Check sheet for the modelled part. Datum: model origin and axes. Units: mm. Face numbers are marked on the shaded views. A direction names the side the tool comes from. Round coordinates to 2 decimals unless told otherwise and drop trailing zeros. Write each loop counter-clockwise with the first axis right and the second up, starting at its lowest first coordinate (ties: lowest second). Pieces come first, ordered by that corner, then holes. Notation, with made-up numbers: (82, 20.5) - (119, 20.5) arc R22 ccw to (119, 29.5) - close; hole circle Ø8 at (-3.5, 30.25). An arc over 180 degrees is marked (long way). Answer as a JSON object with one key per item and string values. Group by question number.
Item 1: Release check for a two-part mould opening along Y. For the marked faces 4, 5 and 6 record: pulls with the +Y half, pulls with the -Y half, needs draft (parallel to the pull), parting line crosses it, or undercut.
Item 2: Sectioned sample at B-B on x = 0. Count the separate pieces of the cut face and the enclosed holes in it, plus the area to 3 significant figures.
Item 3: Sectioned sample at D-D on z = 5.5. Record the boundary of the cut face in (x, y).
Item 4: Thickness scan on line 1 (Y direction, x = 10.5, z = -20.5); line 2 (Y direction, x = 16.5, z = -6); line 3 (X direction, y = 14.5, z = 6.5). Record the ranges inside material, lowest first.
Item 5: Sectioned sample at A-A on y = 22.4. Record the boundary of the cut face in (x, z).
Item 6: Set-up check for the marked faces 1, 2 and 3: record each of +Z, -Z, +X, -X, +Y, -Y from which the full face is reachable in a straight line by a thin tool's end or side.
Item 7: Sectioned sample at C-C on y = 18.5. Record the boundary of the cut face in (x, z), plus the area to 3 significant figures.
Item 8: Gauge pin test, flat ends, axial feed: P1, Ø12, axis at y = -3.5, z = -3, coming from the -X side; P2, Ø4.5, axis at y = 22.4, z = -6, coming from the +X side; P3, Ø1.3, axis at x = 6, y = 15.5, coming from the +Z side; P4, Ø7.5, axis at y = 14, z = 6.5, coming from the -X side. Record the tip position at first contact, or that the pin passes through.
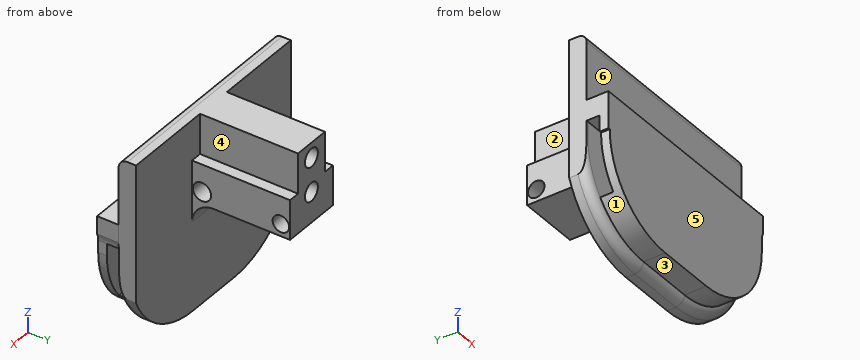
```python
from build123d import *

# Parameters (mm, degrees)
SALIENTE_EXTRUIR1_DEPTH     = 2
SALIENTE_EXTRUIR2_DEPTH     = 24.5
SALIENTE_EXTRUIR3_DEPTH     = 22.5
CORTAR_EXTRUIR1_DEPTH       = 27
CORTAR_EXTRUIR1_DEPTH_BACK  = 65.5
CROQUIS4_R                  = 1.599999999
REDONDEO1_R                 = 3
REDONDEO2_R                 = 5
SALIENTE_EXTRUIR5_START     = 2
SALIENTE_EXTRUIR5_DEPTH     = 2
CROQUIS16_W                 = 2.6
CROQUIS16_H                 = 16.420237112
CORTAR_EXTRUIR8_DEPTH       = 22.5
REDONDEO6_R                 = 2
REDONDEO7_R                 = 2
CROQUIS5_R                  = 2.1
CORTAR_EXTRUIR2_DEPTH       = 20.5
CROQUIS17_R                 = 2.1
CORTAR_EXTRUIR9_DEPTH       = 10
CORTAR_EXTRUIR14_DEPTH      = 11
CORTAR_EXTRUIR14_DEPTH_BACK = 10
CROQUIS18_R                 = 1.9
CROQUIS19_R                 = 18.5
CORTAR_EXTRUIR15_DEPTH      = 3.5
CORTAR_EXTRUIR16_START      = -56
CROQUIS20_R                 = 18.5
CORTAR_EXTRUIR16_DEPTH      = 3.5
CROQUIS21_W                 = 93.525691526
CROQUIS21_H                 = 152.705287602
CROQUIS21_W_2               = 50.201984064
CROQUIS21_H_2               = 74.038187446
CORTAR_EXTRUIR17_DEPTH      = 79
SALIENTE_EXTRUIR6_DEPTH     = 5
CROQUIS23_W                 = 15
CROQUIS23_H                 = 3
CORTAR_EXTRUIR18_DEPTH      = 87


# Read off the part's stored shape, not the designer's step: Saliente-Extruir6
with BuildPart() as part:
    # Croquis1 → Saliente-Extruir1 (new body)
    with BuildSketch(Plane(origin=(0, 0, 0), x_dir=(1, 0, 0), z_dir=(0, 1, 0))):
        with BuildLine():
            Line((-31.5, -9.464532567), (31.5, -9.464532567))
            Line((31.5, -9.464532567), (31.5, 7.964532567))
            ThreePointArc((31.5, 7.964532567), (31.060660172, 9.025192739), (30, 9.464532567))
            Line((30, 9.464532567), (28.160101256, 9.464532567))
            ThreePointArc((28.160101256, 9.464532567), (27.099441084, 9.903872396), (26.660101256, 10.964532567))
            Line((26.660101256, 10.964532567), (26.660101256, 14.266885585))
            ThreePointArc((26.660101256, 14.266885585), (20.802236879, 28.409021208), (6.660101256, 34.266885585))
            Line((6.660101256, 34.266885585), (-6.660101256, 34.266885585))
            ThreePointArc((-6.660101256, 34.266885585), (-20.802236879, 28.409021208), (-26.660101256, 14.266885585))
            Line((-26.660101256, 14.266885585), (-26.660101256, 10.964532567))
            ThreePointArc((-26.660101256, 10.964532567), (-27.099441084, 9.903872396), (-28.160101256, 9.464532567))
            Line((-28.160101256, 9.464532567), (-30, 9.464532567))
            ThreePointArc((-30, 9.464532567), (-31.060660172, 9.025192739), (-31.5, 7.964532567))
            Line((-31.5, 7.964532567), (-31.5, -9.464532567))
        make_face()
    extrude(amount=SALIENTE_EXTRUIR1_DEPTH)

    # Croquis2 → Saliente-Extruir2 (add)
    with BuildSketch(Plane(origin=(0, 0, 0), x_dir=(1, 0, 0), z_dir=(0, 1, 0))):
        Polygon((6.95, -8.819174125), (6.95, -9.464532567), (-6.95, -9.464532567), (-6.95, -8.819174125), (-6.95, 8.819174125), (6.95, 8.819174125), align=None)
    extrude(amount=SALIENTE_EXTRUIR2_DEPTH)

    # Croquis3 → Saliente-Extruir3 (add)
    with BuildSketch(Plane(origin=(0, 2, 0), x_dir=(1, 0, 0), z_dir=(0, 1, 0))):
        with BuildLine():
            ThreePointArc((28.160101256, 9.464532567), (27.375457574, 9.686121721), (26.822638598, 10.285420177))
            Line((26.822638598, 10.285420177), (25.6, 10.285420177))
            Line((25.6, 10.285420177), (25.6, -2.749999823))
            Line((25.6, -2.749999823), (31.5, -2.749999823))
            Line((31.5, -2.749999823), (31.5, 7.964532567))
            ThreePointArc((31.5, 7.964532567), (31.060660172, 9.025192739), (30, 9.464532567))
            Line((30, 9.464532567), (28.160101256, 9.464532567))
        make_face()
        with BuildLine():
            Line((-25.6, 10.285420177), (-26.822638598, 10.285420177))
            ThreePointArc((-26.822638598, 10.285420177), (-27.375457574, 9.686121721), (-28.160101256, 9.464532567))
            Line((-28.160101256, 9.464532567), (-30, 9.464532567))
            ThreePointArc((-30, 9.464532567), (-31.060660172, 9.025192739), (-31.5, 7.964532567))
            Line((-31.5, 7.964532567), (-31.5, -2.749999823))
            Line((-31.5, -2.749999823), (-25.6, -2.749999823))
            Line((-25.6, -2.749999823), (-25.6, 10.285420177))
        make_face()
    extrude(amount=SALIENTE_EXTRUIR3_DEPTH)

    # Croquis4 → Cortar-Extruir1 (cut, two sides: drawn at the far end of the back side and taken through both)
    with BuildSketch(Plane.ZY.offset(25.5).offset(-CORTAR_EXTRUIR1_DEPTH_BACK)):
        with Locations((-6.002353017, 4.3)):
            Circle(CROQUIS4_R)
        with Locations((-6.002353017, 22.4)):
            Circle(CROQUIS4_R)
    extrude(amount=CORTAR_EXTRUIR1_DEPTH + CORTAR_EXTRUIR1_DEPTH_BACK, mode=Mode.SUBTRACT)

    # Redondeo1
    redondeo1_edges = [part.edges().sort_by_distance(p)[0] for p in [
        (28.55, 2, 2.749999823),
    ]]
    fillet(redondeo1_edges, radius=REDONDEO1_R)

    # Redondeo2
    redondeo2_edges = [part.edges().sort_by_distance(p)[0] for p in [
        (0, 2, -8.819174125),
    ]]
    fillet(redondeo2_edges, radius=REDONDEO2_R)

    # Croquis15 → Saliente-Extruir5 (add)
    with BuildSketch(Plane.XZ.offset(SALIENTE_EXTRUIR5_START)):
        with BuildLine():
            Line((-31.5, 9.464532567), (31.5, 9.464532567))
            Line((31.5, 9.464532567), (31.5, -7.489095092))
            ThreePointArc((31.5, -7.489095092), (30.914213562, -8.903308654), (29.5, -9.489095092))
            Line((29.5, -9.489095092), (28.660101256, -9.489095092))
            ThreePointArc((28.660101256, -9.489095092), (27.245887693, -10.074881529), (26.660101256, -11.489095092))
            Line((26.660101256, -11.489095092), (26.660101256, -14.266885585))
            ThreePointArc((26.660101256, -14.266885585), (20.802236879, -28.409021208), (6.660101256, -34.266885585))
            Line((6.660101256, -34.266885585), (1.137553535, -34.266885585))
            Line((1.137553535, -34.266885585), (-1.137553535, -34.266885585))
            Line((-1.137553535, -34.266885585), (-6.660101256, -34.266885585))
            ThreePointArc((-6.660101256, -34.266885585), (-20.802236879, -28.409021208), (-26.660101256, -14.266885585))
            Line((-26.660101256, -14.266885585), (-26.660101256, -11.489095092))
            ThreePointArc((-26.660101256, -11.489095092), (-27.245887693, -10.074881529), (-28.660101256, -9.489095092))
            Line((-28.660101256, -9.489095092), (-29.5, -9.489095092))
            ThreePointArc((-29.5, -9.489095092), (-30.914213562, -8.903308654), (-31.5, -7.489095092))
            Line((-31.5, -7.489095092), (-31.5, 9.464532567))
        make_face()
    extrude(amount=-SALIENTE_EXTRUIR5_DEPTH)

    # Croquis16 → Cortar-Extruir8 (cut)
    with BuildSketch(Plane(origin=(0, 24.5, 0), x_dir=(1, 0, 0), z_dir=(0, 1, 0))):
        with Locations((5.65, -8.484535845)):
            Rectangle(CROQUIS16_W, CROQUIS16_H)
        with Locations((-5.65, -8.484535845)):
            Rectangle(CROQUIS16_W, CROQUIS16_H)
    extrude(amount=-CORTAR_EXTRUIR8_DEPTH, mode=Mode.SUBTRACT)

    # Redondeo6
    redondeo6_edges = [part.edges().sort_by_distance(p)[0] for p in [
        (-31.5, -2, 0.987718738),
        (-30.914213562, -2, -8.903308654),
        (-29.080050628, -2, -9.489095092),
        (-27.245887693, -2, -10.074881529),
        (-26.660101256, -2, -12.877990338),
        (-20.802236879, -2, -28.409021208),
        (0, -2, -34.266885585),
        (20.802236879, -2, -28.409021208),
        (26.660101256, -2, -12.877990338),
        (27.245887693, -2, -10.074881529),
        (29.080050628, -2, -9.489095092),
        (30.914213562, -2, -8.903308654),
        (31.5, -2, 0.987718738),
    ]]
    fillet(redondeo6_edges, radius=REDONDEO6_R - 0.0001)  # a hair under: the kernel refuses the full size

    # Redondeo7
    redondeo7_edges = [part.edges().sort_by_distance(p)[0] for p in [
        (0, -2, 9.464532567),
        (30.914242852, -1.414242852, 9.464532567),
        (-30.914242852, -1.414242852, 9.464532567),
        (31.5, 0.99995, 9.464532567),
        (-31.5, 0.99995, 9.464532567),
    ]]
    fillet(redondeo7_edges, radius=REDONDEO7_R - 0.0001)  # a hair under: the kernel refuses the full size

    # Croquis5 → Cortar-Extruir2 (cut)
    with BuildSketch(Plane(origin=(0, 24.5, 0), x_dir=(1, 0, 0), z_dir=(0, 1, 0))):
        with Locations(Location((0, 1.798301608, 0), (0, 0, 270))):
            Circle(CROQUIS5_R)
        with Locations(Location((0, -6.026932469, 0), (0, 0, 270))):
            Circle(CROQUIS5_R)
        with Locations(Location((-28.55, 1.798301608, 0), (0, 0, 270))):
            Circle(CROQUIS5_R)
        with Locations(Location((28.55, 1.798301608, 0), (0, 0, 270))):
            Circle(CROQUIS5_R)
    extrude(amount=-CORTAR_EXTRUIR2_DEPTH, mode=Mode.SUBTRACT)

    # Croquis17 → Cortar-Extruir9 (cut, symmetric)
    with BuildSketch(Plane(origin=(0, 0, 0), x_dir=(0, 0, -1), z_dir=(1, 0, 0))):
        with Locations((6.002353017, 4.3)):
            Circle(CROQUIS17_R)
    extrude(amount=CORTAR_EXTRUIR9_DEPTH, both=True, mode=Mode.SUBTRACT)

    # Croquis18 → Cortar-Extruir14 (cut, two sides: drawn at the far end of the back side and taken through both)
    with BuildSketch(Plane(origin=(0, 0, 0), x_dir=(0, 0, -1), z_dir=(1, 0, 0)).offset(-CORTAR_EXTRUIR14_DEPTH_BACK)):
        with Locations(Location((6.002353017, 22.4, 0), (0, 0, 180))):
            Circle(CROQUIS18_R)
    extrude(amount=CORTAR_EXTRUIR14_DEPTH + CORTAR_EXTRUIR14_DEPTH_BACK, mode=Mode.SUBTRACT)

    # Croquis19 → Cortar-Extruir15 (cut)
    with BuildSketch(Plane(origin=(31.5, 0, 0), x_dir=(0, 0, -1), z_dir=(1, 0, 0))):
        with Locations((25.179802512, 14.045485316)):
            Circle(CROQUIS19_R)
    extrude(amount=-CORTAR_EXTRUIR15_DEPTH, mode=Mode.SUBTRACT)

    # Croquis20 → Cortar-Extruir16 (cut)
    with BuildSketch(Plane(origin=(28, 0, 0), x_dir=(0, 0, -1), z_dir=(1, 0, 0)).offset(CORTAR_EXTRUIR16_START)):
        with Locations((25.179802512, 14.045485316)):
            Circle(CROQUIS20_R)
    extrude(amount=-CORTAR_EXTRUIR16_DEPTH, mode=Mode.SUBTRACT)

    # Croquis21 → Cortar-Extruir17 (cut)
    with BuildSketch(Plane(origin=(0, 24.5, 0), x_dir=(1, 0, 0), z_dir=(0, 1, 0))):
        Rectangle(CROQUIS21_W, CROQUIS21_H)
        Rectangle(CROQUIS21_W_2, CROQUIS21_H_2, mode=Mode.SUBTRACT)
    extrude(amount=-CORTAR_EXTRUIR17_DEPTH, mode=Mode.SUBTRACT)

    # Saliente-Extruir6 outline → Saliente-Extruir6 (add)
    with BuildSketch(Plane.XZ.offset(2)):
        with BuildLine():
            Line((25.004354391, -5.79015449), (-25.100992032, -5.79015449))
            Line((-25.100992032, -5.79015449), (-25.100992032, -14.266885585))
            Line((-25.100992032, -14.266885585), (-24.660101256, -14.266885585))
            ThreePointArc((-24.660101256, -14.266885585), (-19.388023317, -26.994807646), (-6.660101256, -32.266885585))
            Line((-6.660101256, -32.266885585), (6.660101256, -32.266885585))
            ThreePointArc((6.660101256, -32.266885585), (19.388023317, -26.994807646), (24.660101256, -14.266885585))
            Line((24.660101256, -14.266885585), (24.660101256, -11.489095092))
            ThreePointArc((24.660101256, -11.489095092), (24.747110874, -10.659332312), (25.004354391, -9.865668204))
            Line((25.004354391, -9.865668204), (25.004354391, -5.79015449))
        make_face()
    extrude(amount=SALIENTE_EXTRUIR6_DEPTH)

    # Croquis23 → Cortar-Extruir18 (cut)
    with BuildSketch(Plane(origin=(24.660101256, 0, 0), x_dir=(0, 0, -1), z_dir=(1, 0, 0))):
        with Locations((18.051411886, -3.5)):
            Rectangle(CROQUIS23_W, CROQUIS23_H)
    extrude(amount=-CORTAR_EXTRUIR18_DEPTH, mode=Mode.SUBTRACT)


solid = part.part
```
Completed:
{
 "1": {"face 4": "needs draft", "face 5": "pulls with the -Y half", "face 6": "undercut"},
 "2": {"separate pieces": "1", "enclosed holes": "3", "area": "480 mm²"},
 "3": {"outline": "(-25.1, -2) - (25.1, -2) - (25.1, 2) - (4.35, 2) - (4.35, 24.5) - (2.03, 24.5) - (2.03, 4) - (-2.03, 4) - (-2.03, 24.5) - (-4.35, 24.5) - (-4.35, 2) - (-25.1, 2) - close"},
 "4": {"line 1": "-7 to -5, -2 to 2", "line 2": "-7 to 2", "line 3": "-4.35 to -2.05, 2.05 to 4.35"},
 "5": {"outline": "(-6.95, -8.82) - (6.95, -8.82) - (6.95, -7.9) - (-6.95, -7.9) - close; (-6.95, -4.1) - (6.95, -4.1) - (6.95, 0.27) - (4.35, 0.27) - (4.35, 9.46) - (-4.35, 9.46) - (-4.35, 0.27) - (-6.95, 0.27) - close; hole circle Ø4.2 at (0, -1.8); hole circle Ø4.2 at (0, 6.03)"},
 "6": {"face 1": "-Z, -X, -Y", "face 2": "+Z, -X, +Y", "face 3": "-Z, +X, -X, -Y"},
 "7": {"outline": "(-6.95, -8.82) - (6.95, -8.82) - (6.95, 0.27) - (4.35, 0.27) - (4.35, 9.46) - (-4.35, 9.46) - (-4.35, 0.27) - (-6.95, 0.27) - close; hole circle Ø4.2 at (0, -1.8); hole circle Ø4.2 at (0, 6.03)", "area": "179 mm²"},
 "8": {"P1": "x = -25.1", "P2": "x = 6.95", "P3": "z = 0.27", "P4": "x = -4.35"}
}
